The model under review builds one solid part; all positions refer to its coordinate system, in mm. Face numbers are marked on the shaded views. Coordinates: 2 decimals unless noted, no trailing zeros. Write each loop counter-clockwise with the first axis right and the second up, starting at its lowest first coordinate (ties: lowest second). Pieces come first, ordered by that corner, then holes. Notation, with made-up numbers: (-9, 53.25) - (11, 53.25) arc R22 ccw to (11, 59.25) - close; hole circle Ø10 at (85.25, 43). An arc over 180 degrees is marked (long way). Put each result on its own line as item: value. Start each with the question number.
Item 1: To check wall thickness, follow L1, parallel to X at y = 0, z = -41; L2, parallel to Z at x = 0.5, y = -24; L3, parallel to Z at x = -20, y = -6. State the ranges of each line that lie inside material, in increasing order. Write a range as [from, to].
Item 2: Consider section A-A on z = -20.5. Give the boundary of the cut face in (x, y).
Item 3: For pin 1 (12 mm diameter, centred on x = 15.5, z = -47.5, fed in from -Y); pin 2 (9 mm diameter, centred on x = 0, y = 0, fed in from +Z); pin 3 (4 mm diameter, centred on x = 24.5, z = -68, fed in from +Y); pin 4 (12 mm diameter, centred on y = -7.5, z = -19.5, fed in from -X), all flat-tipped, find the tip position at first contact; note any pin that passes through.
Item 4: Mouldability with a two-part tool opening along Z and no side actions: class the marked faces 1, 2 and 3 as pulls with the +Z half, pulls with the -Z half, needs draft (parallel to the pull), parting line crosses it, or undercut.
Item 5: Consider section B-B on z = -64. Give the boundary of the cut face in (x, y), then the cut area to 3 significant figures.
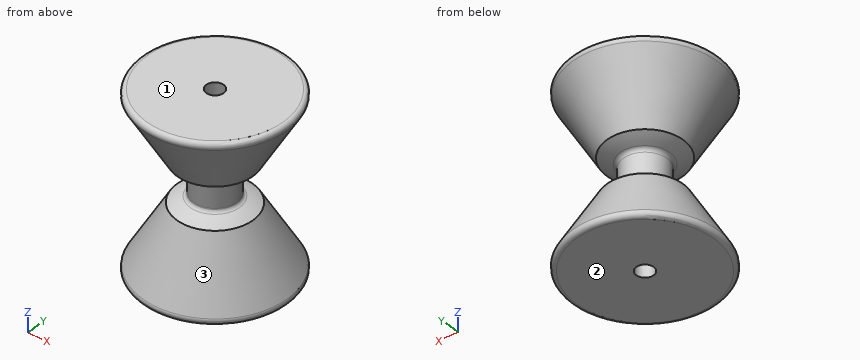
Autodesk Inventor part; units mm, degrees
ref_plane "YZ Plane" through (0, 0, 0) normal (1, 0, 0) x (0, 1, 0)
ref_plane "XZ Plane" through (0, 0, 0) normal (0, 1, 0) x (-1, 0, 0)
ref_plane "XY Plane" through (0, 0, 0) normal (0, 0, 1) x (1, 0, 0)
sketch "Sketch1" plane through (0, 0, 0) normal (0, 1, 0) x (-1, 0, 0)
  line L0 (0, 0) -> (-31.5359, 0)
  line L1 (0, 0) -> (27.4991, 0) construction
  line L2 (-33.2679, -3) -> (-17.5, -30.3109)
  line L3 (-35, 0) -> (8.6719, 0) construction
  line L4 (0, 0) -> (0, -35)
  arc A0 (-17.5, -30.3109) -> (-11.3514, -33.1081) centre (0, 0) ccw
  line L5 (-10, -35) -> (-10, -45.3109)
  line L6 (0, -45.3109) -> (0, -30.3109)
  line L7 (0, -80) -> (-31.5359, -80)
  line L8 (-33.2679, -77) -> (-17.5, -49.6891)
  line L9 (-35, -80) -> (8.6719, -80) construction
  line L10 (0, -80) -> (0, -45)
  arc A1 (-11.3514, -46.8919) -> (-17.5, -49.6891) centre (0, -80) ccw
  line L11 (-10.0944, -45.6071) -> (-10, -45.3109)
  line L12 (0, -45.3109) -> (0, -49.6891)
  arc A2 (-31.5359, 0) -> (-33.2679, -3) centre (-31.5359, -2) ccw
  arc A3 (-33.2679, -77) -> (-31.5359, -80) centre (-31.5359, -78) ccw
  arc A4 (-10, -35) -> (-11.3514, -33.1081) centre (-12, -35) ccw
  arc A5 (-11.3514, -46.8919) -> (-10.0944, -45.6071) centre (-12, -45) ccw
  line L13 (-4, 0) -> (-4, -80)
  dimension "d0" = 35
  dimension "d3" = 60
  dimension "d5" = 10
  dimension "d7" = 2
  dimension "d8" = 80
revolve "Revolution1" add sketch "Sketch1" angle 360 about axis through (0, 0, 0) along (0, 0, -1) contours L13 L7 A3 L8 A1 A5 L11 L5 A4 A0 L2 A2 L0
ref_plane "Work Plane1" through (0, 0, -40) normal (0, 0, 1) x (1, 0, 0)
properties part number "wheel"
Report:
1. L1: [-10, -4], [4, 10]
1. L2: [-80, -60.96], [-19.04, 0]
1. L3: [-80, -55.54], [-24.46, 0]
2. outline: circle Ø46.33 at (0, 0); hole circle Ø8 at (0, 0)
3. pin 1: y = -14.92
3. pin 2: z = 0
3. pin 3: y = 17.41
3. pin 4: x = -26.44
4. face 1: pulls with the +Z half
4. face 2: pulls with the -Z half
4. face 3: undercut
5. outline: circle Ø51.52 at (0, 0); hole circle Ø8 at (0, 0)
5. area: 2,030 mm²
